For this review, use the dimensioned drawing (mm, ordinates from the lowest corner) and the shaded views. A direction names the side the tool comes from. Give positions to 0.01 mm unless a question says otherwise; leave off trailing zeros. Write each loop counter-clockwise with the first axis right and the second up, starting at its lowest first coordinate (ties: lowest second). Pieces come first, ordered by that corner, then holes. Notation, with made-up numbers: (-8, 50) -> (28, 50) arc R17 cw to (28, 82) -> close; hole circle Ø4 at (53, 41.25). An arc over 180 degrees is marked (long way). Write each question's results on one line, items separated by ' | '. Start each with the question number.
(1) Take a section at C-C (z = 69.5). State the section outline as (x, y) points, plus the area to 3 significant figures.
(2) For the marked faces 1, 2 and 3, list the 3-axis set-ups (+Z, -Z, +X, -X, +Y, -Y) from which the entire face can be reached by the end or side of a thin tool; tool diameter is ignored.
(3) Take a section at B-B (y = 80). State the section outline as (x, z) points.
(4) Take a section at A-A (x = 300). State the section outline as (y, z) points.
(5) Clearance check with flat-ended pins moving along their axes: pin 1 (12 mm diameter, centred on y = 136.5, z = 44.5, fed in from +X); pin 2 (1 mm diameter, centred on y = 110.5, z = 45, fed in from -X); pin 3 (6 mm diameter, centred on y = 89, z = 14, fed in from +X). State where each tip first meets the part, or that it passes through.
(6) Take a section at D-D (x = 103). State the section outline as (y, z) points.
(7) To check wall thickness, follow probe 1 along X at (y, z) = (141.5, 152); probe 2 along Z at (x, y) = (198, 150); probe 3 along X at (y, z) = (100, 86.5). State the ranges of each line that lie inside material, in increasing order.
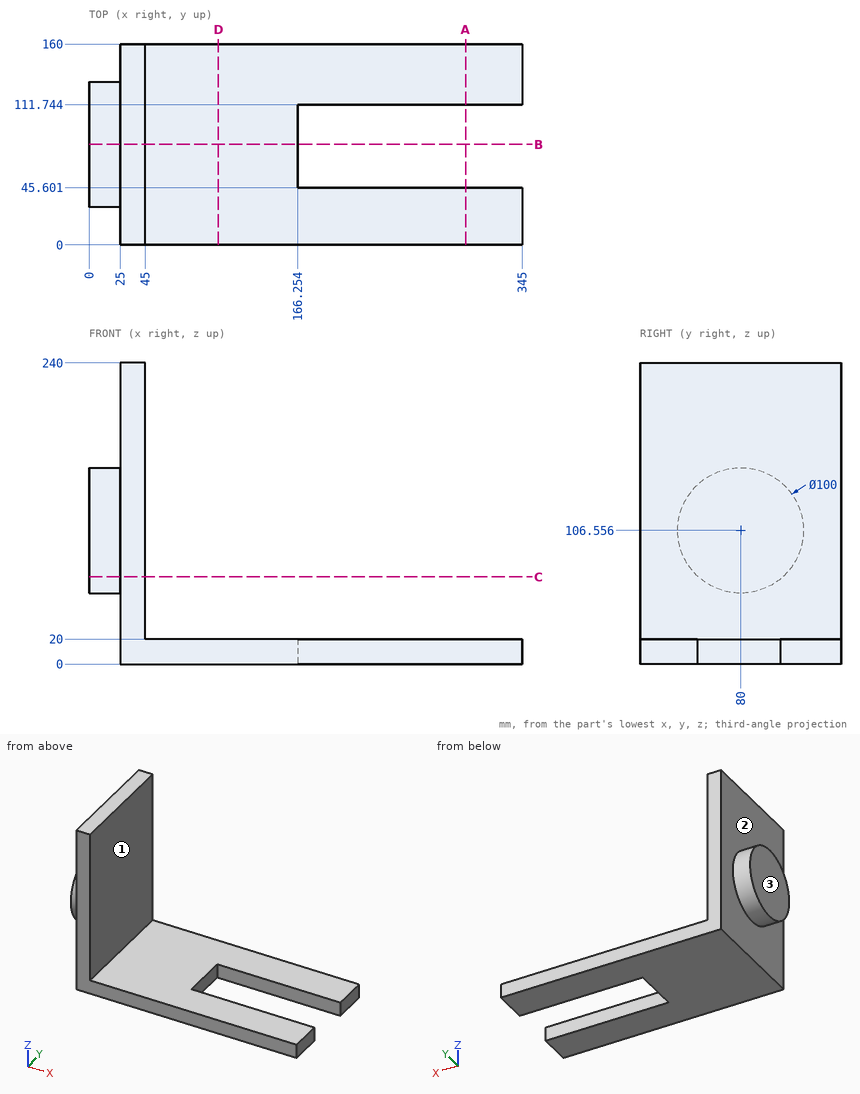
Report:
1) outline: (0, 46.43) -> (25, 46.43) -> (25, 0) -> (45, 0) -> (45, 160) -> (25, 160) -> (25, 113.57) -> (0, 113.57) -> close | area: 4,880 mm2
2) face 1: +Z, +X, +Y, -Y | face 2: -X | face 3: +Z, -Z, -X, +Y, -Y
3) outline: (0, 56.56) -> (25, 56.56) -> (25, 0) -> (166.25, 0) -> (166.25, 20) -> (45, 20) -> (45, 240) -> (25, 240) -> (25, 156.56) -> (0, 156.56) -> close
4) outline: (0, 0) -> (45.6, 0) -> (45.6, 20) -> (0, 20) -> close; (111.74, 0) -> (160, 0) -> (160, 20) -> (111.74, 20) -> close
5) pin 1: x = 45 | pin 2: x = 25 | pin 3: x = 166.25
6) outline: (0, 0) -> (160, 0) -> (160, 20) -> (0, 20) -> close
7) probe 1: 25 to 45 | probe 2: 0 to 20 | probe 3: 0 to 45
